Design review of the part shown in the three views and the two pictorial views. Dimensions are in mm from the part's minimum x, y and z. A direction names the side the tool comes from. Round coordinates to 2 decimals unless told otherwise and drop trailing zeros. Write each loop counter-clockwise with the first axis right and the second up, starting at its lowest first coordinate (ties: lowest second). Pieces come first, ordered by that corner, then holes. Notation, with made-up numbers: (22.5, 55) -> (30.5, 55) arc R25 cw to (30.5, 94) -> close; hole circle Ø4 at (29.5, 51). An arc over 180 degrees is marked (long way). Answer as a JSON object with one key per item and string values. Group by question number.
1) Mouldability with a two-part tool opening along Y and no side actions: class the marked faces 1, 2, 3 and 4 as pulls with the +Y half, pulls with the -Y half, needs draft (parallel to the pull), parting line crosses it, or undercut.
2) We need section C-C, the plane y = 3. Write out the cut boundary in (x, z), then the cut area to 3 significant figures.
3) To check wall thickness, follow probe 1 along Y at (x, z) = (1.2, 6); probe 2 along Y at (x, z) = (6.75, 8.5); probe 3 along Y at (x, z) = (1.5, 8.5). State the ranges of each line that lie inside material, in increasing order. Write a range as [from, to].
4) We need section D-D, the plane z = 3. Write out the cut boundary in (x, y).
5) We need section A-A, the plane x = 6. Write out the cut boundary in (y, z).
6) We need section B-B, the plane z = 6. Write out the cut boundary in (x, y), then the cut area to 3 significant figures.
7) Machinability: for the marked faces 5, 6, 7 and 8, which of the approach directions +Z, -Z, +X, -X, +Y, -Y give a long, thin tool a straight path to every point of the face, cutting with its end or side? Answer none if there is none.
8) Insertion check: pin 1 Ø5 at (y, z) = (2.5, 8) entering from +X; pin 2 Ø4 at (x, z) = (14, 3.5) entering from +Y; pin 3 Ø6 at (x, y) = (5.5, 7) entering from -Z; pin 4 Ø1.5 at (x, z) = (6, 2) entering from -Y. Each pin has a flat end and moves straight along its axis. Give the tip position at first contact, or say it passes through.
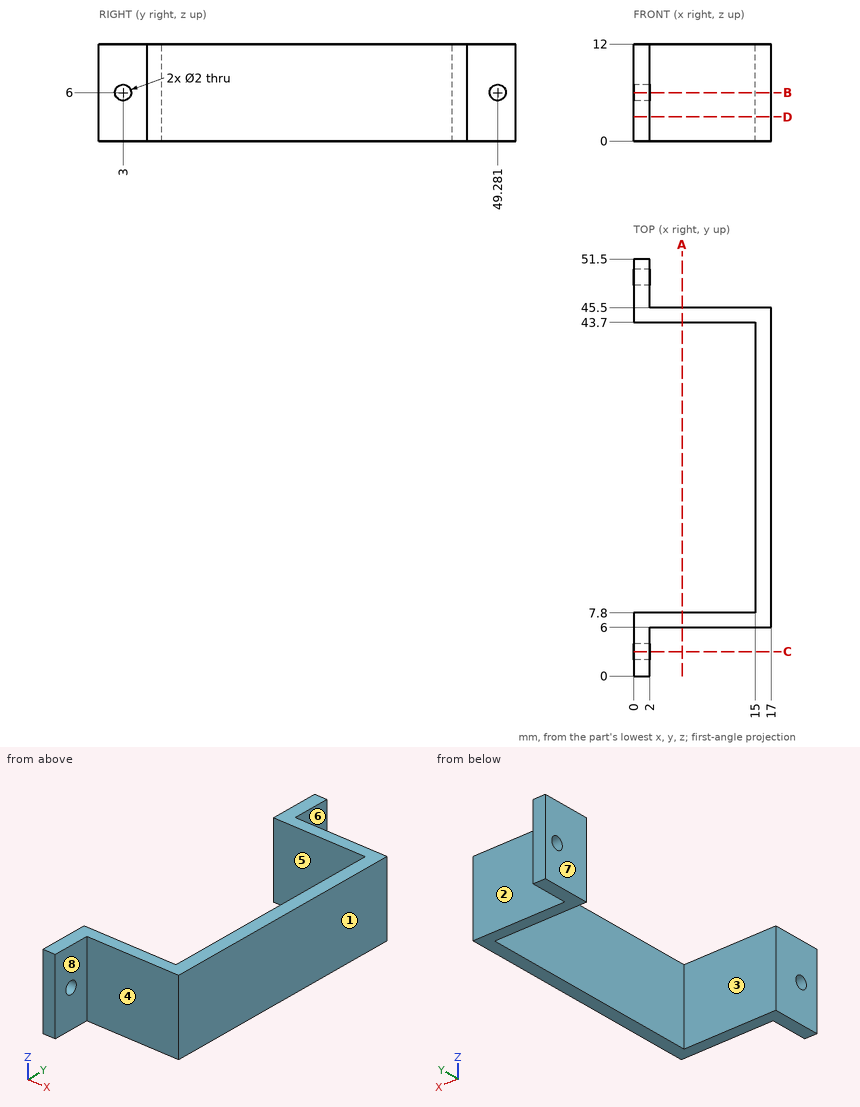
Here are the results:
{
 "1": {"face 1": "needs draft", "face 2": "pulls with the +Y half", "face 3": "undercut", "face 4": "pulls with the -Y half"},
 "2": {"outline": "(0, 0) -> (2, 0) -> (2, 5) -> (0, 5) -> close; (0, 7) -> (2, 7) -> (2, 12) -> (0, 12) -> close", "area": "20.0 mm^2"},
 "3": {"probe 1": "y = [0, 2], [4, 7.8], [43.7, 48.28], [50.28, 51.5]", "probe 2": "y = [6, 7.8], [43.7, 45.5]", "probe 3": "y = [0, 7.8], [43.7, 51.5]"},
 "4": {"outline": "(0, 0) -> (2, 0) -> (2, 6) -> (17, 6) -> (17, 45.5) -> (2, 45.5) -> (2, 51.5) -> (0, 51.5) -> (0, 43.7) -> (15, 43.7) -> (15, 7.8) -> (0, 7.8) -> close"},
 "5": {"outline": "(6, 0) -> (7.8, 0) -> (7.8, 12) -> (6, 12) -> close; (43.7, 0) -> (45.5, 0) -> (45.5, 12) -> (43.7, 12) -> close"},
 "6": {"outline": "(0, 0) -> (2, 0) -> (2, 2) -> (0, 2) -> close; (0, 4) -> (2, 4) -> (2, 6) -> (17, 6) -> (17, 45.5) -> (2, 45.5) -> (2, 48.28) -> (0, 48.28) -> (0, 43.7) -> (15, 43.7) -> (15, 7.8) -> (0, 7.8) -> close; (0, 50.28) -> (2, 50.28) -> (2, 51.5) -> (0, 51.5) -> close", "area": "149 mm^2"},
 "7": {"face 5": "+Z, -Z, -X", "face 6": "+Z, -Z, +X, +Y", "face 7": "+Z, -Z, -X, +Y, -Y", "face 8": "+Z, -Z, +X, -Y"},
 "8": {"pin 1": "stops at x = 2", "pin 2": "stops at y = 45.5", "pin 3": "stops at z = 0", "pin 4": "stops at y = 6"}
}
